Read the model definition and answer for the solid it produces. Units are mm, in the model's axes. A direction names the side the tool comes from. Coordinates: 2 decimals unless noted, no trailing zeros. Loops run counter-clockwise (first coordinate to the right, second up) from the corner with the lowest first, then second, coordinate; pieces in that order, holes last.
from build123d import *

# Parameters (mm, degrees)
F0_W         = 31
F0_H         = 31
F1_DEPTH     = 3
F2_R         = 1.5
F3_DEPTH     = 3
F4_W         = 12.5
F4_H         = 16.75
F5_DEPTH     = 20
F6_W         = 10.5
F6_H         = 14.75
F7_DEPTH     = 23
F8_R         = 20
F9_DEPTH     = 25
F10_W        = 12.5
F10_H        = 1
F11_DEPTH    = 3
F12_T1_DEPTH = 10.5
F13_W        = 12.5
F13_H        = 1
F14_DEPTH    = 3
F15_T1_DEPTH = 10.5


# Not quite as in the source:
# - a fillet or chamfer that OpenCascade refuses, or shapes differently, is made with other operations: its cross-section is extruded or revolved along the edge and cut away or added


with BuildPart() as f1:
    # F0 (on Front) → F1 (new body)
    with BuildSketch(Plane.XZ):
        Rectangle(F0_W, F0_H)
    extrude(amount=F1_DEPTH)

    # F2 (on face) → F3 (cut)
    with BuildSketch(Plane.XZ.offset(3)):
        with Locations((-11.75, -11.75)):
            Circle(F2_R)
        with Locations((-11.75, 11.75)):
            Circle(F2_R)
        with Locations((11.75, 11.75)):
            Circle(F2_R)
        with Locations((11.75, -11.75)):
            Circle(F2_R)
    extrude(amount=-F3_DEPTH, mode=Mode.SUBTRACT)

    # F4 (on face) → F5 (join)
    with BuildSketch(Plane.XZ.offset(3)):
        Rectangle(F4_W, F4_H)
    extrude(amount=F5_DEPTH)

    # F6 (on face) → F7 (cut)
    with BuildSketch(Plane.XZ.offset(23)):
        Rectangle(F6_W, F6_H)
    extrude(amount=-F7_DEPTH, mode=Mode.SUBTRACT)

    # F8 (on face) → F9 (cut)
    with BuildSketch(Plane.YZ.offset(6.25)):
        with Locations((-34, 8.3282930885)):
            Circle(F8_R)
    extrude(amount=-F9_DEPTH, mode=Mode.SUBTRACT)

    # F10 (on face) → F11 (join)
    with BuildSketch(Plane.XZ.offset(3)):
        with Locations((0, -0.5)):
            Rectangle(F10_W, F10_H)
    extrude(amount=-F11_DEPTH)

    # F12: fillet of radius 5 on 1 edges, made by hand

    # F12_s2 → F12_t1 (cut)
    with BuildSketch(Plane.YZ.offset(-5.25)):
        with BuildLine():
            ThreePointArc((0, -1), (-1.5811388301, -0.7434164903), (-3, 0))
            Line((-3, 0), (-3, -1))
            Line((-3, -1), (0, -1))
        make_face()
    extrude(amount=F12_T1_DEPTH, mode=Mode.SUBTRACT)

    # F13 (on face) → F14 (join)
    with BuildSketch(Plane.XZ.offset(3)):
        with Locations((0, 0.5)):
            Rectangle(F13_W, F13_H)
    extrude(amount=-F14_DEPTH)

    # F15: fillet of radius 5 on 1 edges, made by hand

    # F15_s2 → F15_t1 (cut)
    with BuildSketch(Plane.YZ.offset(-5.25)):
        with BuildLine():
            ThreePointArc((-3, 0), (-1.5811388301, 0.7434164903), (0, 1))
            Line((0, 1), (-3, 1))
            Line((-3, 1), (-3, 0))
        make_face()
    extrude(amount=F15_T1_DEPTH, mode=Mode.SUBTRACT)


solid = f1.part
Item 1: A cutting plane is placed at A-A on x = 11.75. Determine the outline of the cut face in (y, z), then the cut area to 3 significant figures.
Numbers:
outline: (-3, -15.5) - (0, -15.5) - (0, -13.25) - (-3, -13.25) - close; (-3, -10.25) - (0, -10.25) - (0, 10.25) - (-3, 10.25) - close; (-3, 13.25) - (0, 13.25) - (0, 15.5) - (-3, 15.5) - close
area: 75.0 mm2
Item 2: A cutting plane is placed at C-C on z = 11.75. Determine the outline of the cut face in (x, y), then the cut area to 3 significant figures.
Numbers:
outline: (-15.5, -3) - (-13.25, -3) - (-13.25, 0) - (-15.5, 0) - close; (-10.25, -3) - (10.25, -3) - (10.25, 0) - (-10.25, 0) - close; (13.25, -3) - (15.5, -3) - (15.5, 0) - (13.25, 0) - close
area: 75.0 mm2
Item 3: Given pin 1 (1.5 mm diameter, centred on x = -3, z = 10.5, fed in from -Y); pin 2 (12 mm diameter, centred on y = -15.5, z = 0.5, fed in from -X); pin 3 (7.5 mm diameter, centred on y = -15.5, z = 3, fed in from +X); pin 4 (1.8 mm diameter, centred on x = 11.75, z = -11.75, fed in from -Y), each flat-ended and moving along its own axis, determine where each tip first touches the part or whether it passes through.
Numbers:
pin 1: stops at y = -3
pin 2: stops at x = -6.25
pin 3: stops at x = 6.25
pin 4: passes through
Item 4: Which of the six approach directions +Z, -Z, +X, -X, +Y, -Y give full straight-line access (tool end or side, diameter ignored) to faces 4 (the face through (0, -11, -7.375)), 5 (the face through (15.5, -1, 0)), 6 (the face through (0, 0, 0)), 7 (the face through (-0.07, -1.56, -0.75)), 8 (the face through (-6.25, -11, -2))?
Numbers:
face 4: +Y, -Y
face 5: +Z, -Z, +X, +Y, -Y
face 6: +Z, -Z, +X, -X, +Y
face 7: -Y
face 8: +Z, -Z, -X, -Y
Item 5: Determine the mould class of faces 1 (the face through (10.56, -1.52, -12.66)), 2 (the face through (6.25, -11, -2)), 3 (the face through (0, -1, 15.5)) for opening direction Z: released by +Z, released by -Z, zero draft, split by the parting line, or undercut.
Numbers:
face 1: undercut
face 2: zero draft
face 3: released by +Z
Item 6: A cutting plane is placed at B-B on y = -9. Determine the outline of the cut face in (x, z) (3 decimals).
Numbers:
outline: (-6.25, -8.375) - (6.25, -8.375) - (6.25, 8.375) - (-6.25, 8.375) - close; hole (-5.25, -7.375) - (5.25, -7.375) - (5.25, 7.375) - (-5.25, 7.375) - close
Item 7: Find the intervals of material crossed by line 1 along Z through (x, y) = (-11.75, -0.8); line 2 along X through (y, z) = (-11, -6); line 3 along Z through (x, y) = (4, -10.75) (3 decimals), in increasing order.
Numbers:
line 1: z = -15.5 to -13.25, -10.25 to 10.25, 13.25 to 15.5
line 2: x = -6.25 to -5.25, 5.25 to 6.25
line 3: z = -8.375 to -7.375, 7.375 to 8.375
Item 8: A cutting plane is placed at D-D on z = 6.5. Determine the outline of the cut face in (x, y).
Numbers:
outline: (-15.5, -3) - (-6.25, -3) - (-6.25, -14.08) - (-5.25, -14.08) - (-5.25, 0) - (-15.5, 0) - close; (5.25, -14.08) - (6.25, -14.08) - (6.25, -3) - (15.5, -3) - (15.5, 0) - (5.25, 0) - close
